Part model, mm, in its own coordinate system. Coordinates: 2 decimals unless noted, no trailing zeros. Write each loop counter-clockwise with the first axis right and the second up, starting at its lowest first coordinate (ties: lowest second). Pieces come first, ordered by that corner, then holes. Notation, with made-up numbers: (63.25, -2) - (90.25, -2) arc R28 cw to (90.25, 17) - close; hole circle Ø1 at (1, -21.75). An arc over 180 degrees is marked (long way). Use a Markdown table: item, result.
```python
from build123d import *

# Parameters (mm, degrees)
SKETCH1_R           = 12
SKETCH1_R_2         = 8
BOSS_EXTRUDE1_DEPTH = 3
CHAMFER1_SIZE       = 0.5
SKETCH2_R           = 10.95
SKETCH2_R_2         = 9.05
CUT_EXTRUDE1_DEPTH  = 2


with BuildPart() as part:
    # Sketch1 → Boss-Extrude1 (new body)
    with BuildSketch(Plane.XY):
        Circle(SKETCH1_R)
        Circle(SKETCH1_R_2, mode=Mode.SUBTRACT)
    extrude(amount=BOSS_EXTRUDE1_DEPTH)

    # Chamfer1
    chamfer1_edges = [part.edges().sort_by_distance(p)[0] for p in [
        (-12, 0, 0),
        (-12, 0, 3),
        (-8, 0, 0),
        (-8, 0, 3),
    ]]
    chamfer(chamfer1_edges, length=CHAMFER1_SIZE)

    # Sketch2 → Cut-Extrude1 (cut)
    with BuildSketch(Plane.XY.offset(3)):
        Circle(SKETCH2_R)
        Circle(SKETCH2_R_2, mode=Mode.SUBTRACT)
    extrude(amount=-CUT_EXTRUDE1_DEPTH, mode=Mode.SUBTRACT)


solid = part.part
```
Item 1: Band-saw the part on A-A, the plane y = 0. Give the cut face in (x, z), then the cut area to 3 significant figures.
From the geometry:
| item | result |
|---|---|
| outline | (-12, 0.5) - (-11.5, 0) - (-8.5, 0) - (-8, 0.5) - (-8, 2.5) - (-8.5, 3) - (-9.05, 3) - (-9.05, 1) - (-10.95, 1) - (-10.95, 3) - (-11.5, 3) - (-12, 2.5) - close; (8, 0.5) - (8.5, 0) - (11.5, 0) - (12, 0.5) - (12, 2.5) - (11.5, 3) - (10.95, 3) - (10.95, 1) - (9.05, 1) - (9.05, 3) - (8.5, 3) - (8, 2.5) - close |
| area | 15.4 mm^2 |
Item 2: Drop a flat-ended pin along its axis: P1, Ø1.5, axis at x = -4.5, z = 2, coming from the +Y side. Give the stop position or say it passes through.
From the geometry:
| item | result |
|---|---|
| P1 | y = 11.4 |
Item 3: Band-saw the part on C-C, the plane z = 2.05. Give the cut face in (x, y), then the cut area to 3 significant figures.
From the geometry:
| item | result |
|---|---|
| outline | circle Ø24 at (0, 0); circle Ø18.1 at (0, 0); hole circle Ø21.9 at (0, 0); hole circle Ø16 at (0, 0) |
| area | 132 mm^2 |
Item 4: Drill centre lines: probe 1 along Y at (x, z) = (0, 2.2); probe 2 along Y at (x, z) = (0, 2.55); probe 3 along X at (y, z) = (-4.25, 2.15). Where is each one in solid material? Low to high.
From the geometry:
| item | result |
|---|---|
| probe 1 | -12 to -10.95, -9.05 to -8, 8 to 9.05, 10.95 to 12 |
| probe 2 | -11.95 to -10.95, -9.05 to -8.05, 8.05 to 9.05, 10.95 to 11.95 |
| probe 3 | -11.22 to -10.09, -7.99 to -6.78, 6.78 to 7.99, 10.09 to 11.22 |
Item 5: Two-plate mould, pull along X, no slides. Class faces 1 (the face through (-1.73, -7.81, 1.49)), 2 (the face through (-11.99, 0.53, 1.49)), 3 (the face through (-4, -8, 0)): pulls with the +X half, pulls with the -X half, needs draft (parallel to the pull), parting line crosses it, or undercut.
From the geometry:
| item | result |
|---|---|
| face 1 | undercut |
| face 2 | parting line crosses it |
| face 3 | needs draft |
